Design review of the part built by this model. Coordinates are the model's own, in mm. A direction names the side the tool comes from. Give positions to 0.01 mm unless a question says otherwise; leave off trailing zeros. Loops run counter-clockwise (first coordinate to the right, second up) from the corner with the lowest first, then second, coordinate; pieces in that order, holes last. Notation, with made-up numbers: M 61.25,-26.5 L 92.25,-26.5 A24 ccw 92.25,8.5 Z; hole C 87.25,-4.75 d7. An arc over 180 degrees is marked long. Answer as CSV lines item,"result".
```python
from build123d import *

# Parameters (mm, degrees)
SKETCH1_W           = 32.4
SKETCH1_H           = 30
SKETCH1_R           = 1.75
BOSS_EXTRUDE1_DEPTH = 25
SKETCH2_R           = 4
CUT_EXTRUDE1_DEPTH  = 20
BOSS_EXTRUDE2_START = 3
SKETCH3_W           = 32.4
SKETCH3_H           = 30
SKETCH3_R           = 4
BOSS_EXTRUDE2_DEPTH = 3
BOSS_EXTRUDE3_START = 23.5
SKETCH4_W           = 32.4
SKETCH4_H           = 30
BOSS_EXTRUDE3_DEPTH = 23.5
SKETCH5_R           = 1.25
CUT_EXTRUDE2_DEPTH  = 2.45
SKETCH6_W           = 22
SKETCH6_H           = 4
CUT_EXTRUDE3_DEPTH  = 5.15


with BuildPart() as part:
    # Sketch1 → Boss-Extrude1 (new body)
    with BuildSketch(Plane(origin=(0, 0, 0), x_dir=(1, 0, 0), z_dir=(0, 1, 0))):
        with Locations((16.2, -15)):
            Rectangle(SKETCH1_W, SKETCH1_H)
        with Locations(Location((6.2, -5, 0), (0, 0, 270))):
            Circle(SKETCH1_R, mode=Mode.SUBTRACT)
        with Locations(Location((26.2, -5, 0), (0, 0, 270))):
            Circle(SKETCH1_R, mode=Mode.SUBTRACT)
        with Locations(Location((26.2, -25, 0), (0, 0, 270))):
            Circle(SKETCH1_R, mode=Mode.SUBTRACT)
        with Locations(Location((6.2, -25, 0), (0, 0, 270))):
            Circle(SKETCH1_R, mode=Mode.SUBTRACT)
    extrude(amount=BOSS_EXTRUDE1_DEPTH)

    # Sketch2 → Cut-Extrude1 (cut)
    with BuildSketch(Plane(origin=(0, 25, 0), x_dir=(1, 0, 0), z_dir=(0, 1, 0))):
        with Locations(Location((16.2, -15, 0), (0, 0, 270))):
            Circle(SKETCH2_R)
    extrude(amount=-CUT_EXTRUDE1_DEPTH, mode=Mode.SUBTRACT)

    # Sketch3 → Boss-Extrude2 (add)
    with BuildSketch(Plane(origin=(0, 25, 0), x_dir=(1, 0, 0), z_dir=(0, 1, 0)).offset(BOSS_EXTRUDE2_START)):
        with Locations((16.2, -15)):
            Rectangle(SKETCH3_W, SKETCH3_H)
        with BuildLine():
            ThreePointArc((11, -2), (8.656854249, -7.656854249), (3, -10))
            Line((3, -10), (3, -2))
            Line((3, -2), (11, -2))
        make_face(mode=Mode.SUBTRACT)
        with BuildLine():
            ThreePointArc((29.4, -10), (23.743145751, -7.656854249), (21.4, -2))
            Line((21.4, -2), (29.4, -2))
            Line((29.4, -2), (29.4, -10))
        make_face(mode=Mode.SUBTRACT)
        with BuildLine():
            ThreePointArc((21.4, -28), (23.743145751, -22.343145751), (29.4, -20))
            Line((29.4, -20), (29.4, -28))
            Line((29.4, -28), (21.4, -28))
        make_face(mode=Mode.SUBTRACT)
        with BuildLine():
            ThreePointArc((3, -20), (8.656854249, -22.343145751), (11, -28))
            Line((11, -28), (3, -28))
            Line((3, -28), (3, -20))
        make_face(mode=Mode.SUBTRACT)
        with Locations(Location((16.2, -15, 0), (0, 0, 270))):
            Circle(SKETCH3_R, mode=Mode.SUBTRACT)
    extrude(amount=-BOSS_EXTRUDE2_DEPTH)

    # Sketch4 → Boss-Extrude3 (add)
    with BuildSketch(Plane(origin=(0, 28, 0), x_dir=(1, 0, 0), z_dir=(0, 1, 0)).offset(BOSS_EXTRUDE3_START)):
        with Locations((16.2, -15)):
            Rectangle(SKETCH4_W, SKETCH4_H)
        with BuildLine():
            Line((5.15, -20.294320277), (5.15, -9.705679723))
            ThreePointArc((5.15, -9.705679723), (4.085025855, -9.926078406), (3, -10))
            Line((3, -10), (3, -2))
            Line((3, -2), (11, -2))
            ThreePointArc((11, -2), (10.996832804, -2.225089113), (10.987333723, -2.45))
            Line((10.987333723, -2.45), (21.412666277, -2.45))
            ThreePointArc((21.412666277, -2.45), (21.403167196, -2.225089113), (21.4, -2))
            Line((21.4, -2), (29.4, -2))
            Line((29.4, -2), (29.4, -10))
            ThreePointArc((29.4, -10), (28.314974145, -9.926078406), (27.25, -9.705679723))
            Line((27.25, -9.705679723), (27.25, -20.294320277))
            ThreePointArc((27.25, -20.294320277), (28.314974145, -20.073921594), (29.4, -20))
            Line((29.4, -20), (29.4, -28))
            Line((29.4, -28), (21.4, -28))
            ThreePointArc((21.4, -28), (21.403167196, -27.774910887), (21.412666277, -27.55))
            Line((21.412666277, -27.55), (10.987333723, -27.55))
            ThreePointArc((10.987333723, -27.55), (10.996832804, -27.774910887), (11, -28))
            Line((11, -28), (3, -28))
            Line((3, -28), (3, -20))
            ThreePointArc((3, -20), (4.085025855, -20.073921594), (5.15, -20.294320277))
        make_face(mode=Mode.SUBTRACT)
    extrude(amount=-BOSS_EXTRUDE3_DEPTH)

    # Sketch5 → Cut-Extrude2 (cut)
    with BuildSketch(Plane(origin=(0, 0, 0), x_dir=(-1, 0, 0), z_dir=(0, 0, -1))):
        with Locations((-22.2, 49)):
            Circle(SKETCH5_R)
        with Locations((-10.2, 34)):
            Circle(SKETCH5_R)
    extrude(amount=-CUT_EXTRUDE2_DEPTH, mode=Mode.SUBTRACT)

    # Sketch6 → Cut-Extrude3 (cut)
    with BuildSketch(Plane.ZY):
        with Locations((15, 30)):
            Rectangle(SKETCH6_W, SKETCH6_H)
    extrude(amount=-CUT_EXTRUDE3_DEPTH, mode=Mode.SUBTRACT)


solid = part.part
```
1. We need section D-D, the plane y = 16.5. Write out the cut boundary in (x, z), plus the area to 3 significant figures.
Answer block:
outline,"M 0,0 L 32.4,0 L 32.4,30 L 0,30 Z; hole C 6.2,5 d3.5; hole C 6.2,25 d3.5; hole C 16.2,15 d8; hole C 26.2,5 d3.5; hole C 26.2,25 d3.5"
area,"883 mm²"
2. We need section C-C, the plane z = 5. Write out the cut boundary in (x, y).
Answer block:
outline,"M 0,0 L 4.45,0 L 4.45,25 L 3,25 L 3,28 L 0,28 Z; M 0,32 L 3,32 L 3,51.5 L 0,51.5 Z; M 7.95,0 L 24.45,0 L 24.45,25 L 21.98,25 L 21.98,28 L 10.42,28 L 10.42,25 L 7.95,25 Z; M 27.95,0 L 32.4,0 L 32.4,51.5 L 29.4,51.5 L 29.4,25 L 27.95,25 Z"
3. We need section A-A, the plane y = 34. Write out the cut boundary in (x, z), plus the area to 3 significant figures.
Answer block:
outline,"M 0,0 L 8.95,0 L 8.95,2 L 3,2 L 3,10 A8 cw 5.15,9.71 L 5.15,20.29 A8 cw 3,20 L 3,28 L 11,28 A8 cw 10.99,27.55 L 21.41,27.55 A8 cw 21.4,28 L 29.4,28 L 29.4,20 A8 cw 27.25,20.29 L 27.25,9.71 A8 cw 29.4,10 L 29.4,2 L 21.4,2 A8 cw 21.41,2.45 L 11.45,2.45 L 11.45,0 L 32.4,0 L 32.4,30 L 0,30 Z"
area,"334 mm²"
4. For faces 3 (the cylindrical face through (6.28, 12.32, 23.25)), 4 (the flat face through (29.4, 38, 6)), 5 (the flat face through (1, 30, 4)), list the 3-axis set-ups (+Z, -Z, +X, -X, +Y, -Y) from which the entire face can be reached by the end or side of a thin tool; tool diameter is ignored.
Answer block:
face 3,"+Y, -Y"
face 4,"+Y"
face 5,"-X"
5. To check wall thickness, follow L1, parallel to X at y = 7, z = 5; L2, parallel to Z at x = 26, y = 14; L3, parallel to Z at x = 26, y = 40. State the ranges of each line that lie inside material, in increasing order. Write a range as [from, to].
Answer block:
L1,"[0, 4.45], [7.95, 24.45], [27.95, 32.4]"
L2,"[0, 3.26], [6.74, 23.26], [26.74, 30]"
L3,"[0, 2], [28, 30]"
6. We need section B-B, the plane x = 26.2. Write out the cut boundary in (y, z).
Answer block:
outline,"M 0,0 L 51.5,0 L 51.5,2 L 25,2 L 25,3.25 L 0,3.25 Z; M 0,6.75 L 25,6.75 L 25,9.33 L 28,9.33 L 28,20.67 L 25,20.67 L 25,23.25 L 0,23.25 Z; M 0,26.75 L 25,26.75 L 25,28 L 51.5,28 L 51.5,30 L 0,30 Z"
7. The part is to be moulded in two halves that separate along Z. For faces 1 (the flat face through (16, 40, 2.45)), 2 (the flat face through (0, 26, 15)), say which applies: pulls with the +Z half, pulls with the -Z half, needs draft (parallel to the pull), parting line crosses it, or undercut.
Answer block:
face 1,"undercut"
face 2,"needs draft"
8. For P1, Ø7.5, axis at x = 14, z = 17, coming from the +Y side; P2, Ø2.5, axis at x = 6.5, z = 6, coming from the +Y side, all flat-tipped, find the tip position at first contact; note any pin that passes through.
Answer block:
P1,"y = 28"
P2,"y = 25"
